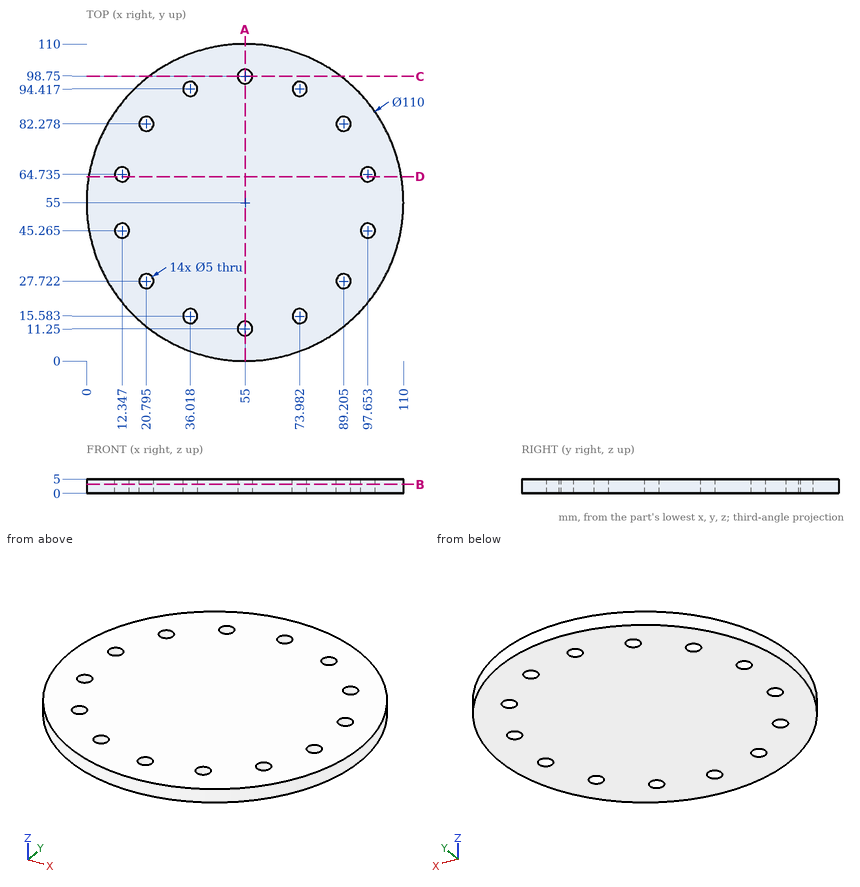
Design review of the part shown in the three views and the two pictorial views. Dimensions are in mm from the part's minimum x, y and z. Give positions to 0.01 mm unless a question says otherwise; leave off trailing zeros. Write each loop counter-clockwise with the first axis right and the second up, starting at its lowest first coordinate (ties: lowest second). Pieces come first, ordered by that corner, then holes. Notation, with made-up numbers: M 12,43.5 L 49,43.5 A19 ccw 49,55.5 Z; hole C 52.25,-39.5 d2. An arc over 180 degrees is marked long. Answer as CSV lines item,"result".
1. Wall thickness on line 1 (Y direction, x = 99, z = 1.4); line 2 (Y direction, x = 95.5, z = 2) (1 decimal); line 3 (X direction, y = 45.5, z = 2.45) (1 decimal): over which ranges is each line inside the solid? List them lowest first.
Findings:
line 1,"y = 22 to 43.16, 47.37 to 62.63, 66.84 to 88"
line 2,"y = 17.8 to 44, 46.5 to 63.5, 66 to 92.2"
line 3,"x = 0.8 to 9.9, 14.8 to 95.2, 100.1 to 109.2"
2. Consider section B-B, the plane z = 3.15. Count the separate pieces of the cut face and the enclosed holes in it, then the cut area to 3 significant figures.
Findings:
separate pieces,"1"
enclosed holes,"14"
area,"9,230 mm2"
3. Consider section C-C, the plane y = 98.75. Write out the cut boundary in (x, z), then the cut area to 3 significant figures.
Findings:
outline,"M 21.67,0 L 52.5,0 L 52.5,5 L 21.67,5 Z; M 57.5,0 L 88.33,0 L 88.33,5 L 57.5,5 Z"
area,"308 mm2"
4. For pin 1 (8 mm diameter, centred on x = 97.65, y = 64.74, fed in from +Z); pin 2 (4.5 mm diameter, centred on x = 12.35, y = 45.26, fed in from +Z); pin 3 (1.5 mm diameter, centred on x = 16.5, z = 1, fed in from -Y); pin 4 (1 mm diameter, centred on x = 63.5, z = 3.5, fed in from +Y) (1 decimal), all flat-tipped, find the tip position at first contact; note any pin that passes through.
Findings:
pin 1,"stops at z = 5"
pin 2,"passes through"
pin 3,"stops at y = 15"
pin 4,"stops at y = 109.4"
5. Consider section D-D, the plane y = 64. Write out the cut boundary in (x, z), then the cut area to 3 significant figures.
Findings:
outline,"M 0.74,0 L 9.96,0 L 9.96,5 L 0.74,5 Z; M 14.74,0 L 95.26,0 L 95.26,5 L 14.74,5 Z; M 100.04,0 L 109.26,0 L 109.26,5 L 100.04,5 Z"
area,"495 mm2"
6. Consider section A-A, the plane x = 55. Write out the cut boundary in (y, z).
Findings:
outline,"M 0,0 L 8.75,0 L 8.75,5 L 0,5 Z; M 13.75,0 L 96.25,0 L 96.25,5 L 13.75,5 Z; M 101.25,0 L 110,0 L 110,5 L 101.25,5 Z"
